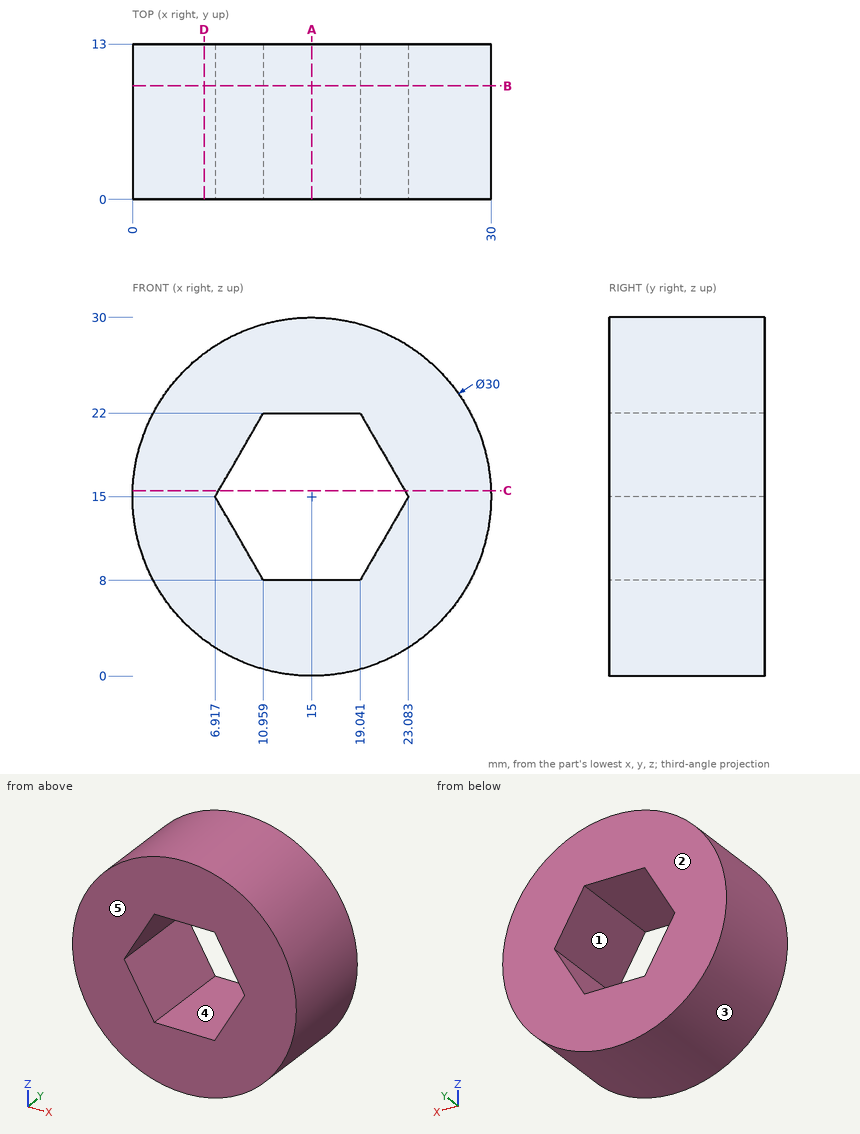
Study the drawing (mm; zero at the part's minimum x, y, z) and answer. A direction names the side the tool comes from. Give positions to 0.01 mm unless a question says otherwise; leave off trailing zeros. Write each loop counter-clockwise with the first axis right and the second up, starting at its lowest first coordinate (ties: lowest second). Pieces come first, ordered by that corner, then holes.
Item 1: Section D-D, the plane x = 6 is taken. Write down the section's boundary in (y, z), plus the area to 3 significant figures.
Item 2: Section B-B, the plane y = 9.5 is taken. Write down the section's boundary in (x, z), plus the area to 3 significant figures.
Item 3: Determine the mould class of the marked faces 1, 2 and 3 for opening direction Z: released by +Z, released by -Z, zero draft, split by the parting line, or undercut.
Item 4: Find the intervals of material crossed by line 1 along X through (y, z) = (6.25, 15); line 2 along Z through (x, y) = (16.5, 8.25) (1 decimal); line 3 along Z through (x, y) = (18.5, 2.5) (1 decimal), in increasing order.
Item 5: Section A-A, the plane x = 15 is taken. Write down the section's boundary in (y, z).
Item 6: Flat-ended cylindrical pins translate along their axes: P1, Ø5, axis at x = 9.5, y = 4.5, coming from the +Z side; P2, Ø2, axis at y = 6.5, z = 26.5, coming from the +X side; P3, Ø5, axis at x = 14.5, y = 5, coming from the +Z side; P4, Ø4, axis at y = 10.5, z = 4, coming from the -X side. Find the tip coordinate at first contact, or state that the pin passes through.
Item 7: Section C-C, the plane z = 15.5 is taken. Write down the section's boundary in (x, y) (1 decimal).
Item 8: Which of the six approach directions +Z, -Z, +X, -X, +Y, -Y give full straight-line access (tool end or side, diameter ignored) to the marked faces 4 and 5?
Completed:
1. outline: (0, 3) - (13, 3) - (13, 27) - (0, 27) - close
1. area: 312 mm2
2. outline: circle Ø30 at (15, 15); hole (6.92, 15) - (10.96, 8) - (19.04, 8) - (23.08, 15) - (19.04, 22) - (10.96, 22) - close
2. area: 537 mm2
3. face 1: undercut
3. face 2: zero draft
3. face 3: split by the parting line
4. line 1: x = 0 to 6.92, 23.08 to 30
4. line 2: z = 0.1 to 8, 22 to 29.9
4. line 3: z = 0.4 to 8, 22 to 29.6
5. outline: (0, 0) - (13, 0) - (13, 8) - (0, 8) - close; (0, 22) - (13, 22) - (13, 30) - (0, 30) - close
6. P1: stops at z = 29.7
6. P2: stops at x = 25.71
6. P3: stops at z = 30
6. P4: stops at x = 3
7. outline: (0, 0) - (7.2, 0) - (7.2, 13) - (0, 13) - close; (22.8, 0) - (30, 0) - (30, 13) - (22.8, 13) - close
8. face 4: +Y, -Y
8. face 5: +Z, -Z, +X, -X, -Y
